Could you check a few things on this model? Use its own coordinates, in mm. A direction names the side the tool comes from. Coordinates: 2 decimals unless noted, no trailing zeros. Write each loop counter-clockwise with the first axis right and the second up, starting at its lowest first coordinate (ties: lowest second). Pieces come first, ordered by that corner, then holes. Notation, with made-up numbers: M -39.5,28 L 13.5,28 A17 cw 13.5,41 Z; hole C -16,64 d11. An arc over 180 degrees is marked long. Answer as CSV lines item,"result". Start each with the question number.
Item 1: Suppose I cut it at A-A, the plane x = 57.5. Write out the boundary of the cut face in (y, z).
Item 2: Suppose I cut it at C-C, the plane y = -189. Write out the boundary of the cut face in (x, z), and give its area (3 significant figures).
Item 3: Suppose I cut it at D-D, the plane x = 60. Write out the boundary of the cut face in (y, z), and give its area (3 significant figures).
Item 4: On a 3-axis mill with a long thin cutter (end or side, diameter ignored), from which of +Z, -Z, +X, -X, +Y, -Y can I reach the whole of each face in a straight line? I mean faces 1 (the flat face through (44.497, -180, 2)), 2 (the flat face through (44.497, -199, 2)), 3 (the cylindrical face through (43.812, -192.234, 3.187)), 4 (the flat face through (47, -189, 0)). Say none if no direction works.
Item 5: I'm going to push flat-ended pins straight in: P1, Ø2, axis at y = -181, z = 1.5, coming from the +X side; P2, Ø2, axis at x = 46, y = -180.5, coming from the -Z side; P3, Ø1.2, axis at x = 52, z = 2.5, coming from the -Y side; P4, Ø5, axis at x = 42.5, y = -189.71, coming from the +Z side. Where does each tip first touch, or does it pass through?
Item 6: Suppose I cut it at B-B, the plane z = 3.6. Write out the boundary of the cut face in (x, y).
Item 7: If I drill on line 1 along X through (y, z) = (-189.5, 0.2); line 2 along X through (y, z) = (-191.75, 2.4); line 3 along X through (y, z) = (-179, 1.8), over which ranges is the centre line in solid material (lowest first)? Write a range as [from, to].
Item 8: We'd pull the mould along Y, two halves only. Please class faces 5 (the flat face through (53, -185.705, 2)), 6 (the flat face through (61.497, -190, 2)), 7 (the cylindrical face through (55.236, -191.44, 3.187)): +Y half, -Y half, draft (parallel to the pull), parting line (faces both ways), or undercut.
```python
from build123d import *

# Parameters (mm, degrees)
CROQUIS2_R              = 1.5
SALIENTE_EXTRUIR1_DEPTH = 4
CROQUIS3_R              = 2.85
CORTAR_EXTRUIR1_DEPTH   = 1.65
CROQUIS4_W              = 4
CROQUIS4_H              = 11
CORTAR_EXTRUIR2_DEPTH   = 2


with BuildPart() as part:
    # Croquis2 → Saliente-Extruir1 (new body)
    with BuildSketch(Plane.XY):
        Polygon((38.497217209, -204.70543153), (46.497217209, -204.70543153), (46.497217209, -193.70543153), (61.497217209, -193.70543153), (61.497217209, -185.70543153), (46.497217209, -185.70543153), (46.497217209, -174.70543153), (38.497217209, -174.70543153), align=None)
        with Locations((42.497217209, -189.70543153)):
            Circle(CROQUIS2_R, mode=Mode.SUBTRACT)
        with Locations((57.497217209, -189.70543153)):
            Circle(CROQUIS2_R, mode=Mode.SUBTRACT)
        with Locations((49.997217209, -189.70543153)):
            Circle(CROQUIS2_R, mode=Mode.SUBTRACT)
    extrude(amount=SALIENTE_EXTRUIR1_DEPTH)

    # Croquis3 → Cortar-Extruir1 (cut)
    with BuildSketch(Plane.XY.offset(4)):
        with Locations((42.497217209, -189.70543153)):
            Circle(CROQUIS3_R)
        with Locations((49.997217209, -189.70543153)):
            Circle(CROQUIS3_R)
        with Locations((57.497217209, -189.70543153)):
            Circle(CROQUIS3_R)
    extrude(amount=-CORTAR_EXTRUIR1_DEPTH, mode=Mode.SUBTRACT)

    # Croquis4 → Cortar-Extruir2 (cut)
    with BuildSketch(Plane(origin=(46.497217209, 0, 0), x_dir=(0, 0, -1), z_dir=(1, 0, 0))):
        with Locations((-2, -199.20543153)):
            Rectangle(CROQUIS4_W, CROQUIS4_H)
        with Locations((-2, -180.20543153)):
            Rectangle(CROQUIS4_W, CROQUIS4_H)
    extrude(amount=-CORTAR_EXTRUIR2_DEPTH, mode=Mode.SUBTRACT)


solid = part.part
```
Ans:
1,outline,"M -193.71,0 L -191.21,0 L -191.21,2.35 L -192.56,2.35 L -192.56,4 L -193.71,4 Z; M -188.21,0 L -185.71,0 L -185.71,4 L -186.86,4 L -186.86,2.35 L -188.21,2.35 Z"
2,outline,"M 38.5,0 L 41.17,0 L 41.17,2.35 L 39.74,2.35 L 39.74,4 L 38.5,4 Z; M 43.82,0 L 48.67,0 L 48.67,2.35 L 47.24,2.35 L 47.24,4 L 45.26,4 L 45.26,2.35 L 43.82,2.35 Z; M 51.32,0 L 56.17,0 L 56.17,2.35 L 54.74,2.35 L 54.74,4 L 52.76,4 L 52.76,2.35 L 51.32,2.35 Z; M 58.82,0 L 61.5,0 L 61.5,4 L 60.26,4 L 60.26,2.35 L 58.82,2.35 Z"
2,area,"46.0 mm^2"
3,outline,"M -193.71,0 L -185.71,0 L -185.71,4 L -188.34,4 L -188.34,2.35 L -191.07,2.35 L -191.07,4 L -193.71,4 Z"
3,area,"27.5 mm^2"
4,face 1,"+Z, -Z, +X, +Y"
4,face 2,"+Z, -Z, +X, -Y"
4,face 3,"+Z"
4,face 4,"-Z, +X, -X, +Y, -Y"
5,P1,"stops at x = 44.5"
5,P2,"passes through"
5,P3,"stops at y = -193.71"
5,P4,"stops at z = 2.35"
6,outline,"M 38.5,-204.71 L 44.5,-204.71 L 44.5,-193.71 L 61.5,-193.71 L 61.5,-185.71 L 44.5,-185.71 L 44.5,-174.71 L 38.5,-174.71 Z; hole C 42.5,-189.71 d5.7; hole C 50,-189.71 d5.7; hole C 57.5,-189.71 d5.7"
7,line 1,"x = [38.5, 41.01], [43.98, 48.51], [51.48, 56.01], [58.98, 61.5]"
7,line 2,"x = [38.5, 40.51], [44.48, 48.01], [51.98, 55.51], [59.48, 61.5]"
7,line 3,"x = [38.5, 44.5]"
8,face 5,"+Y half"
8,face 6,"draft"
8,face 7,"undercut"
